The listing builds one solid part. Answer for the finished solid, in the listing's coordinates (mm). Face numbers are marked on the shaded views. Round coordinates to 2 decimals unless told otherwise and drop trailing zeros. Loops run counter-clockwise (first coordinate to the right, second up) from the corner with the lowest first, then second, coordinate; pieces in that order, holes last. Notation, with made-up numbers: (30.5, 37.5) -> (38.5, 37.5) arc R18 ccw to (38.5, 50.5) -> close; hole circle Ø7 at (6.25, 79.25). An arc over 180 degrees is marked (long way). Use a Markdown table: item, result. Add a question column.
Q1. Given pin 1 Ø0.5 at (x, z) = (6.5, -5.5) entering from -Y; pin 2 Ø0.7 at (x, z) = (-4.5, -3.5) entering from -Y, each flat-ended and moving along its own axis, determine where each tip first touches the part or whether it passes through.
Q2. For a pull along Z with two mould halves and no side action, classify the marked faces 1, 2 and 3 as released by +Z, released by -Z, zero draft, split by the parting line, or undercut.
Q3. Section D-D on z = -2.75 is taken. Give the vertices of the cut face in (x, y).
Q4. Section C-C on x = 7.5 is taken. Give the vertices of the cut face in (y, z), then the cut area to 3 significant figures.
Q5. Section A-A on z = -5.25 is taken. Give the vertices of the cut face in (x, y), then the cut area to 3 significant figures.
Q6. Section B-B on x = 1 is taken. Give the vertices of the cut face in (y, z), then the cut area to 3 significant figures.
Q7. Consider line 1 (X direction, y = -0.95, z = -6); line 2 (Z direction, x = -6.25, y = -1); line 3 (X direction, y = -0.2, z = -4.5). Determine where each line is inside the solid, lowest interval first.
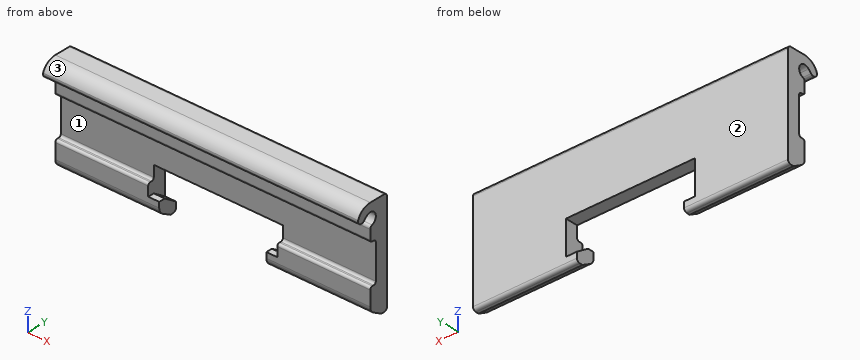
Autodesk Inventor part; units mm, degrees
ref_plane "mitBHZ_XY" through (0, -1.2, -3.9) normal (0, 1, 0) x (1, 0, 0)
ref_plane "mitBHZ_YZ" through (0, -1.2, -3.9) normal (1, 0, 0) x (0, 0, -1)
ref_plane "mitBHZ_ZX" through (0, -1.2, -3.9) normal (0, 0, -1) x (0, 1, 0)
sketch "Sketch_1" plane through (0, 0, 0) normal (1, 0, 0) x (0, 1, 0)
  line L0 (-0.2, 0) -> (-1.2, 0)
  arc A0 (-1.2, 0) -> (-2.0731, -0.5918) centre (-1.2, -0.94) ccw
  arc A1 (-2.0731, -0.5918) -> (-1.6536, -0.8272) centre (-1.83, -0.65) ccw
  line L1 (-1.6536, -0.8272) -> (-1.4822, -0.6565)
  arc A2 (-1.0667, -1.3171) -> (-1.4822, -0.6565) centre (-1.2, -0.94) ccw
  arc A3 (-1.0667, -1.3171) -> (-1.2, -1.5057) centre (-1, -1.5057) ccw
  line L2 (-1.2, -1.5057) -> (-1.2, -2.1)
  arc A4 (-1.2, -2.1) -> (-1.05, -2.25) centre (-1.05, -2.1) ccw
  line L3 (-1.05, -2.25) -> (-0.95, -2.25)
  arc A5 (-0.8, -2.4) -> (-0.95, -2.25) centre (-0.95, -2.4) ccw
  line L4 (-0.8, -2.4) -> (-0.8, -4.6)
  arc A6 (-0.95, -4.75) -> (-0.8, -4.6) centre (-0.95, -4.6) ccw
  line L5 (-0.95, -4.75) -> (-1.05, -4.75)
  arc A7 (-1.05, -4.75) -> (-1.2, -4.9) centre (-1.05, -4.9) ccw
  line L6 (-1.2, -4.9) -> (-1.2, -5.8494)
  arc A8 (-1.2, -5.8494) -> (-0.95, -6.2825) centre (-0.7, -5.8494) ccw
  line L7 (-0.95, -6.2825) -> (-0.4, -6.6)
  line L8 (-0.4, -6.6) -> (-0.2, -6.6)
  arc A9 (-0.2, -6.6) -> (0, -6.4) centre (-0.2, -6.4) ccw
  line L9 (0, -6.4) -> (0, -0.2)
  arc A10 (0, -0.2) -> (-0.2, 0) centre (-0.2, -0.2) ccw
extrude "Extrusion1" add sketch "Sketch_1" along normal mid plane 20
sketch "Sketch_2" plane through (0, 0, 0) normal (0, 1, 0) x (-1, 0, 0)
  line L0 (4.1, -3.9) -> (-4.1, -3.9)
  line L1 (-4.1, -3.9) -> (-4.1, -5.5)
  line L2 (-4.1, -5.5) -> (-3.4, -5.5)
  line L3 (-3.4, -5.5) -> (-3.4, -6.9)
  line L4 (-3.4, -6.9) -> (3.4, -6.9)
  line L5 (3.4, -6.9) -> (3.4, -5.5)
  line L6 (3.4, -5.5) -> (4.1, -5.5)
  line L7 (4.1, -5.5) -> (4.1, -3.9)
extrude "Extrusion2" cut sketch "Sketch_2" against normal blind 2
sketch "Sketch_4" plane through (0, 0, 0) normal (1, 0, 0) x (0, 1, 0)
  line L0 (0.2, -5.3) -> (-1.0965, -5.3)
  line L1 (-1.0965, -5.3) -> (0.2, -6.1745)
  line L2 (0.2, -6.1745) -> (0.2, -5.3)
extrude "Extrusion3" cut sketch "Sketch_4" along normal mid plane 8.2
ref_plane "mitBHZ_XY" through (0, -1.2, -3.9) normal (0, 1, 0) x (1, 0, 0)
ref_plane "mitBHZ_YZ" through (0, -1.2, -3.9) normal (1, 0, 0) x (0, 0, -1)
ref_plane "mitBHZ_ZX" through (0, -1.2, -3.9) normal (0, 0, -1) x (0, 1, 0)
properties part number "ESG 6.6x20 BHZ 1082540000"
Checked values:
| question | item | result |
|---|---|---|
| 1 | pin 1 | stops at y = -1.2 |
| 1 | pin 2 | stops at y = -0.8 |
| 2 | face 1 | undercut |
| 2 | face 2 | zero draft |
| 2 | face 3 | released by +Z |
| 3 | outline | (-10, -0.8) -> (10, -0.8) -> (10, 0) -> (-10, 0) -> close |
| 4 | outline | (-2.07, -0.59) arc R0.25 ccw to (-1.65, -0.83) -> (-1.48, -0.66) arc R0.4 cw (long way) to (-1.07, -1.32) arc R0.2 ccw to (-1.2, -1.51) -> (-1.2, -2.1) arc R0.15 ccw to (-1.05, -2.25) -> (-0.95, -2.25) arc R0.15 cw to (-0.8, -2.4) -> (-0.8, -4.6) arc R0.15 cw to (-0.95, -4.75) -> (-1.05, -4.75) arc R0.15 ccw to (-1.2, -4.9) -> (-1.2, -5.85) arc R0.5 ccw to (-0.95, -6.28) -> (-0.4, -6.6) -> (-0.2, -6.6) arc R0.2 ccw to (0, -6.4) -> (0, -0.2) arc R0.2 ccw to (-0.2, 0) -> (-1.2, 0) arc R0.94 ccw to start |
| 4 | area | 6.96 mm2 |
| 5 | outline | (-10, -1.2) -> (-4.1, -1.2) -> (-4.1, 0) -> (-10, 0) -> close; (4.1, -1.2) -> (10, -1.2) -> (10, 0) -> (4.1, 0) -> close |
| 5 | area | 14.2 mm2 |
| 6 | outline | (-2.07, -0.59) arc R0.25 ccw to (-1.65, -0.83) -> (-1.48, -0.66) arc R0.4 cw (long way) to (-1.07, -1.32) arc R0.2 ccw to (-1.2, -1.51) -> (-1.2, -2.1) arc R0.15 ccw to (-1.05, -2.25) -> (-0.95, -2.25) arc R0.15 cw to (-0.8, -2.4) -> (-0.8, -3.9) -> (0, -3.9) -> (0, -0.2) arc R0.2 ccw to (-0.2, 0) -> (-1.2, 0) arc R0.94 ccw to start |
| 6 | area | 4.26 mm2 |
| 7 | line 1 | x = -10 to -3.4, 3.4 to 10 |
| 7 | line 2 | z = -6.25 to -4.75, -2.25 to -1.29, -0.59 to 0 |
| 7 | line 3 | x = -10 to -4.1, 4.1 to 10 |
